from build123d import *

# Parameters (mm, degrees)
SKETCH1_W             = 11
SKETCH1_H             = 27
BOSS_EXTRUDE1_DEPTH   = 33
SKETCH1_W_2           = 18
BOSS_EXTRUDE1_2_DEPTH = 33
BOSS_EXTRUDE2_DEPTH   = 13
SKETCH1_5_W           = 24
SKETCH1_5_H           = 27
BOSS_EXTRUDE4_DEPTH   = 33
CUT_EXTRUDE1_DEPTH    = 24
CUT_EXTRUDE2_DEPTH    = 12


with BuildPart() as part:
    # Sketch1 → Boss-Extrude1 (new body)
    with BuildSketch(Plane(origin=(0, 0, 0), x_dir=(1, 0, 0), z_dir=(0, 1, 0))):
        with Locations((-5.5, 0)):
            Rectangle(SKETCH1_W, SKETCH1_H)
    extrude(amount=BOSS_EXTRUDE1_DEPTH)

    # Sketch1_3 → Boss-Extrude2 (add)
    with BuildSketch(Plane(origin=(0, 0, 0), x_dir=(1, 0, 0), z_dir=(0, 1, 0))):
        Polygon((-24, 13.5), (-11, 13.5), (-11, -13.5), align=None)
    extrude(amount=BOSS_EXTRUDE2_DEPTH)



with BuildPart() as body_2:
    # Sketch1 → Boss-Extrude1 2 (new body)
    with BuildSketch(Plane(origin=(0, 0, 0), x_dir=(1, 0, 0), z_dir=(0, 1, 0))):
        with Locations((33, 0)):
            Rectangle(SKETCH1_W_2, SKETCH1_H)
    extrude(amount=BOSS_EXTRUDE1_2_DEPTH)


with BuildPart() as part_1:
    add(part.part)

    add(body_2.part)  # Boss-Extrude4 merges body 2
    # Sketch1_5 → Boss-Extrude4 (add)
    with BuildSketch(Plane(origin=(0, 0, 0), x_dir=(1, 0, 0), z_dir=(0, 1, 0))):
        with Locations((12, 0)):
            Rectangle(SKETCH1_5_W, SKETCH1_5_H)
    extrude(amount=BOSS_EXTRUDE4_DEPTH)

    # Sketch3 → Cut-Extrude1 (cut)
    with BuildSketch(Plane.ZY.offset(-24)):
        Polygon((13.5, 33), (-13.5, 33), (-13.5, 21), align=None)
        Polygon((13.5, 0), (13.5, 33), (-1.5, 0), align=None)
    extrude(amount=CUT_EXTRUDE1_DEPTH, mode=Mode.SUBTRACT)

    # Sketch4 → Cut-Extrude2 (cut)
    with BuildSketch(Plane(origin=(42, 0, 0), x_dir=(0, 0, -1), z_dir=(1, 0, 0))):
        Polygon((4.5, 33), (-13.5, 18), (-13.5, 33), align=None)
    extrude(amount=-CUT_EXTRUDE2_DEPTH, mode=Mode.SUBTRACT)


solid = part_1.part
Part model, mm, in its own coordinate system. A direction names the side the tool comes from. Give positions to 0.01 mm unless a question says otherwise; leave off trailing zeros. Loops run counter-clockwise (first coordinate to the right, second up) from the corner with the lowest first, then second, coordinate; pieces in that order, holes last. Notation, with made-up numbers: (-9.75, -13) -> (24.25, -13) arc R27 ccw to (24.25, 5) -> close; hole circle Ø3 at (-12, -13). An arc over 180 degrees is marked (long way). Write each question's results on one line, items separated by ' | '. Start each with the question number.
Q1. Band-saw the part on D-D on z = -6.25. List the corners of the cut face in (x, y).
Q2. Pull direction X, two halves, no side cores. Call faces 1 (the face through (9, 13, -13.5)), 2 (the face through (24, 9, 9)), 3 (the face through (-11, 23, 0)): +X half, -X half, draft (parallel to the pull), parting line (faces both ways), or undercut.
Q3. Wall check: L1, parallel to X at y = 31.5, z = -9.75; L2, parallel to X at y = 19, z = 7; L3, parallel to X at y = 9, z = 12.25. Give the ranges that are in metal, low to high.
Q4. Band-saw the part on C-C on y = 20. List the corners of the cut face in (x, z), plus the area to 3 significant figures.
Q5. Which spindle directions (+Z, -Z, +X, -X, +Y, -Y) get a long thin tool onto all of the face, cutting with end or side? Do faces 4 (the face through (42, 13, 0)), 5 (the face through (30, 29, 8)), 6 (the face through (0, 9, 9)), 7 (the face through (0, 28, -3)), 8 (the face through (-16, 13, -3)). Say none if no direction does.
Q6. Pin check, flat tips, straight feed: P1, Ø3, axis at y = 15.5, z = 4, coming from the -X side; P2, Ø1.5, axis at y = 4, z = 3.5, coming from the -X side; P3, Ø1, axis at y = 11.5, z = 3.5, coming from the -X side; P4, Ø4, axis at y = 29.5, z = 0, coming from the +X side. Stop position of each tip, or through.
Q7. Band-saw the part on A-A on x = 36. List the corners of the cut face in (y, z), plus the area to 3 significant figures.
Q8. Band-saw the part on B-B on z = 11.5. List the corners of the cut face in (x, y), plus the area to 3 significant figures.
Results are:
1) outline: (-20.51, 0) -> (42, 0) -> (42, 33) -> (24, 33) -> (24, 24.22) -> (0, 24.22) -> (0, 33) -> (-11, 33) -> (-11, 13) -> (-20.51, 13) -> close
2) face 1: draft | face 2: undercut | face 3: -X half
3) L1: x = -11 to 0, 24 to 42 | L2: x = -11 to 42 | L3: x = -11.6 to 0, 24 to 42
4) outline: (-11, -13.5) -> (42, -13.5) -> (42, 11.1) -> (30, 11.1) -> (30, 13.5) -> (24, 13.5) -> (24, 7.59) -> (0, 7.59) -> (0, 13.5) -> (-11, 13.5) -> close | area: 1,260 mm²
5) face 4: +Z, -Z, +X, +Y, -Y | face 5: +Z, +X, +Y | face 6: +Z, -Y | face 7: -Z, +Y | face 8: +Z, -Z, -X, +Y
6) P1: stops at x = -11 | P2: stops at x = -16.18 | P3: stops at x = -16.06 | P4: stops at x = 42
7) outline: (0, -13.5) -> (33, -13.5) -> (33, -4.5) -> (18, 13.5) -> (0, 13.5) -> close | area: 756 mm²
8) outline: (-11.96, 0) -> (0, 0) -> (0, 28.6) -> (24, 28.6) -> (24, 0) -> (42, 0) -> (42, 19.67) -> (30, 19.67) -> (30, 33) -> (24, 33) -> (24, 32.11) -> (0, 32.11) -> (0, 33) -> (-11, 33) -> (-11, 13) -> (-11.96, 13) -> close | area: 894 mm²
